CAD build for the part. Positions are in the model's coordinates, mm. Round coordinates to 2 decimals unless told otherwise and drop trailing zeros. Order: outer loops, then holes, each group sorted by start corner. A loop starts at its lowest first (then second) coordinate and runs counter-clockwise, first axis right, second up.
```python
from build123d import *

# Parameters (mm, degrees)
F0_R           = 1.488728542
F1_DEPTH       = 5
F5_D           = 2
F5_CSINK_D     = 2.5
F5_CSINK_ANGLE = 90


# Not quite as in the source:
# - a feature of the source that left no trace in its solid (it failed there, or was rolled back) is left out


with BuildPart() as f1:
    # F0 (on Front) → F1 (new body)
    with BuildSketch(Plane.XZ):
        with BuildLine():
            Line((-6.25, -2.6532969418), (6.25, -2.6532969418))
            ThreePointArc((6.25, -2.6532969418), (5.854172537, 3.0491244048), (0.1517511904, 2.6532969418))
            Line((0.1517511904, 2.6532969418), (-0.1517511904, 2.6532969418))
            ThreePointArc((-0.1517511904, 2.6532969418), (-5.854172537, 3.0491244048), (-6.25, -2.6532969418))
        make_face()
        with Locations((-3.2008755952, 0)):
            Circle(F0_R, mode=Mode.SUBTRACT)
        with Locations((3.2008755952, 0)):
            Circle(F0_R, mode=Mode.SUBTRACT)
    extrude(amount=F1_DEPTH)

    # F5 (through all)
    with Locations(Plane(origin=(0, 0, -2.6532969418), x_dir=(1, 0, 0), z_dir=(0, 0, -1))):
        with Locations((0, 2.525947988)):
            CounterSinkHole(F5_D / 2, F5_CSINK_D / 2, counter_sink_angle=F5_CSINK_ANGLE)


solid = f1.part
```
1. Mould opens along Z. For faces 1 (the face through (-5.786, -2.465, 3.107)), 2 (the face through (3.007, -2.465, 1.476)), 3 (the face through (-3.395, -2.465, 1.476)), 4 (the face through (1, -2.57, 0.53)) say: released by +Z, released by -Z, zero draft, split by the parting line, or undercut.
2. Cut at A-A, the plane x = 0. Write the cut outline in (y, z).
3. Cut at D-D, the plane z = 1.25. Write the cut outline in (x, y).
4. Cut at B-B, the plane z = 0. Write the cut outline in (x, y), and give its area (3 significant figures).
5. Cut at C-C, the plane y = -0.7. Write the cut outline in (x, z), and give its area (3 significant figures).
6. Pin check, flat tips, straight feed: P1, Ø1.5, axis at y = -2, z = 1, coming from the -X side; P2, Ø2, axis at x = 5, y = -3.5, coming from the +Z side; P3, Ø2, axis at y = -1, z = 3, coming from the -X side. Stop position of each tip, or through.
7. Drill centre lines: line 1 (X direction, y = -3, z = -0.5); line 2 (X direction, y = -3.95, z = 1); line 3 (X direction, y = -4.6, z = -1.25). Where is each one in solid material? Low to high.
Outcome:
1. face 1: split by the parting line
1. face 2: undercut
1. face 3: undercut
1. face 4: zero draft
2. outline: (-5, -2.65) - (-3.78, -2.65) - (-3.53, -2.4) - (-3.53, 2.65) - (-5, 2.65) - close; (-1.53, -2.4) - (-1.28, -2.65) - (0, -2.65) - (0, 2.65) - (-1.53, 2.65) - close
3. outline: (-7.04, -5) - (-4.01, -5) - (-4.01, 0) - (-7.04, 0) - close; (-2.39, -5) - (2.39, -5) - (2.39, 0) - (-2.39, 0) - close; (4.01, -5) - (7.04, -5) - (7.04, 0) - (4.01, 0) - close; hole circle Ø2 at (0, -2.53)
4. outline: (-7.24, -5) - (-4.69, -5) - (-4.69, 0) - (-7.24, 0) - close; (-1.71, -5) - (1.71, -5) - (1.71, 0) - (-1.71, 0) - close; (4.69, -5) - (7.24, -5) - (7.24, 0) - (4.69, 0) - close; hole circle Ø2 at (0, -2.53)
4. area: 39.5 mm2
5. outline: (-6.25, -2.65) - (6.25, -2.65) arc R4.04 ccw to (0.15, 2.65) - (-0.15, 2.65) arc R4.04 ccw to start; hole circle Ø2.98 at (-3.2, 0); hole circle Ø2.98 at (3.2, 0)
5. area: 71.4 mm2
6. P1: stops at x = -7.24
6. P2: stops at z = 3.96
6. P3: stops at x = -6.71
7. line 1: x = -7.21 to -4.6, -1.8 to -0.88, 0.88 to 1.8, 4.6 to 7.21
7. line 2: x = -7.12 to -4.3, -2.1 to 2.1, 4.3 to 7.12
7. line 3: x = -7.04 to -4.01, -2.39 to 2.39, 4.01 to 7.04
